The figure shows three views and two pictorial views of one solid part (mm, origin at its lowest corner). Answer the questions. Coordinates: 2 decimals unless noted, no trailing zeros. Write each loop counter-clockwise with the first axis right and the second up, starting at its lowest first coordinate (ties: lowest second). Pieces come first, ordered by that corner, then holes.
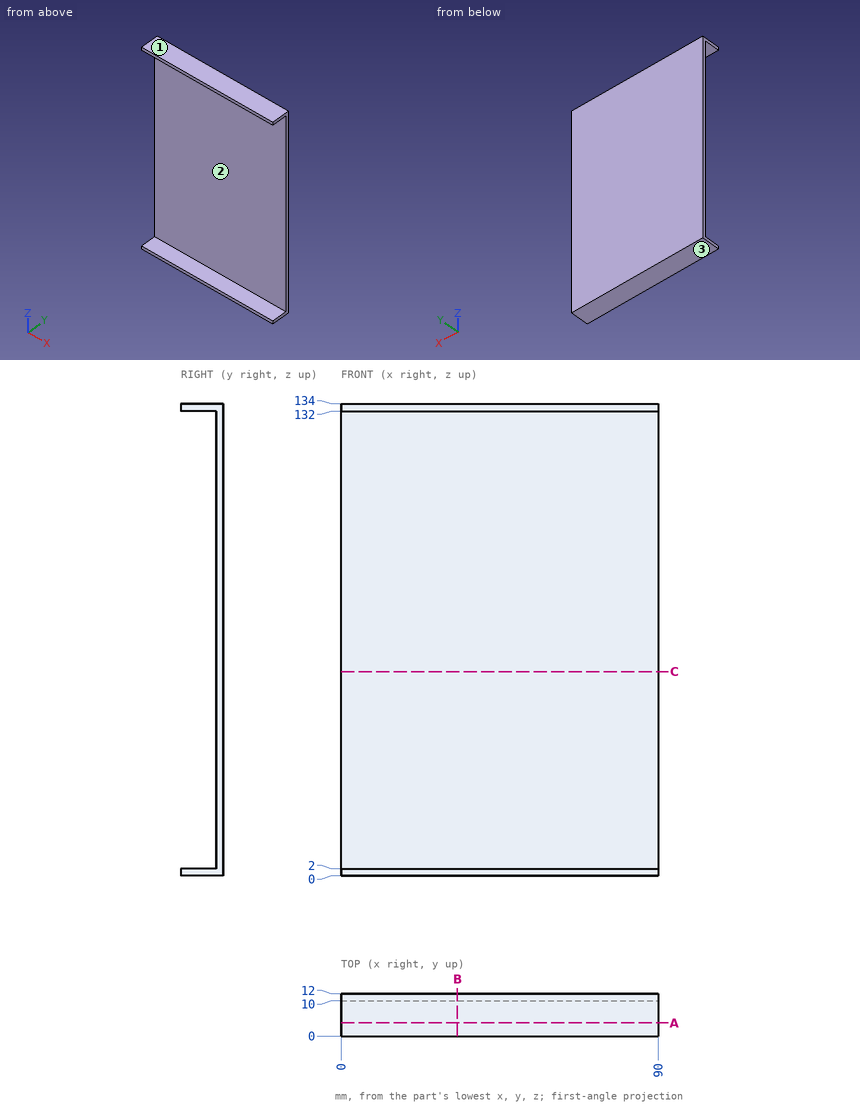
1. A flat-ended cylindrical pin translates along its axis: P1, Ø1.5, axis at x = 44, z = 77, coming from the -Y side. Find the tip coordinate at first contact, or state that the pin passes through.
Results found:
P1: stops at y = 10
2. Find the intervals of material crossed by L1, parallel to Z at x = 72, y = 6.25; L2, parallel to Y at x = 21, z = 56, in increasing order.
Results found:
L1: z = 0 to 2, 132 to 134
L2: y = 10 to 12
3. Section C-C on z = 58 is taken. Give the vertices of the cut face in (x, y), then the cut area to 3 significant figures.
Results found:
outline: (0, 10) - (90, 10) - (90, 12) - (0, 12) - close
area: 180 mm2
4. Section B-B on x = 33 is taken. Give the vertices of the cut face in (y, z).
Results found:
outline: (0, 0) - (12, 0) - (12, 134) - (0, 134) - (0, 132) - (10, 132) - (10, 2) - (0, 2) - close
5. Section A-A on y = 3.75 is taken. Give the vertices of the cut face in (x, z), then the cut area to 3 significant figures.
Results found:
outline: (0, 0) - (90, 0) - (90, 2) - (0, 2) - close; (0, 132) - (90, 132) - (90, 134) - (0, 134) - close
area: 360 mm2
6. For a pull along Z with two mould halves and no side action, classify the marked faces 1, 2 and 3 as pulls with the +Z half, pulls with the -Z half, needs draft (parallel to the pull), parting line crosses it, or undercut.
Results found:
face 1: pulls with the +Z half
face 2: undercut
face 3: pulls with the -Z half
